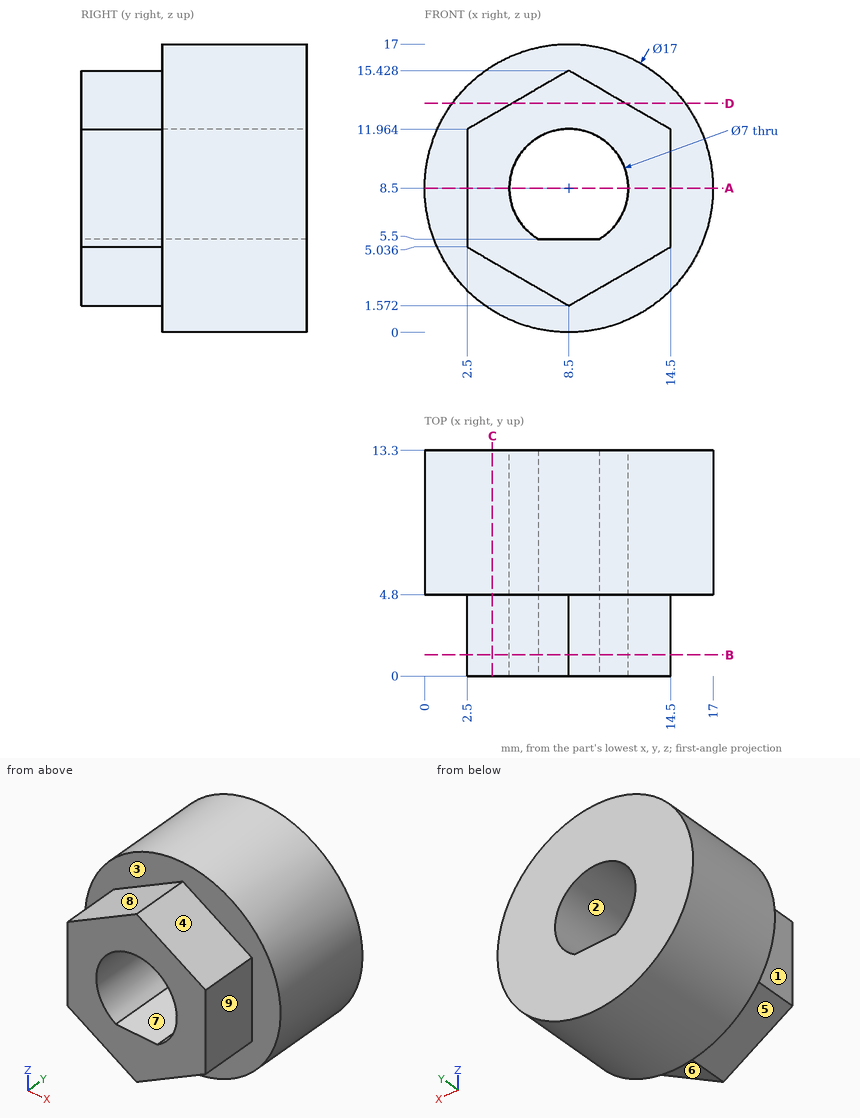
Study the drawing (mm; zero at the part's minimum x, y, z) and answer. A direction names the side the tool comes from. Coordinates: 2 decimals unless noted, no trailing zeros. Loops run counter-clockwise (first coordinate to the right, second up) from the corner with the lowest first, then second, coordinate; pieces in that order, holes last. Notation, with made-up numbers: (55, 85.5) -> (66, 85.5) arc R21 cw to (66, 120.5) -> close; hole circle Ø7 at (0.5, 19). An arc over 180 degrees is marked (long way). Write each question's results on one line, items separated by ' | '. Start each with the question number.
1) Find section C-C on x = 4. Determine the outline of the cut face in (y, z).
2) Find section B-B on y = 1.25. Determine the outline of the cut face in (x, z).
3) Find section D-D on z = 13.5. Determine the outline of the cut face in (x, y), then the cut area to 3 significant figures.
4) Flat-ended cylindrical pins translate along their axes: P1, Ø1.4, axis at y = 3, z = 8, coming from the -X side; P2, Ø1.4, axis at y = 2.5, z = 9.5, coming from the +X side; P3, Ø5, axis at y = 5.5, z = 15, coming from the -X side. Find the tip coordinate at first contact, or state that the pin passes through.
5) The mould has two halves that part along X. Classify the marked faces 1, 2, 3 and 4: pulls with the +X half, pulls with the -X half, needs draft (parallel to the pull), parting line crosses it, or undercut.
6) For the marked faces 5, 6, 7, 8 and 9, determine the directions among +Z, -Z, +X, -X, +Y, -Y from which every point of the face is accessible in a straight line to the end or side of a thin tool.
7) Find section A-A on z = 8.5. Determine the outline of the cut face in (x, y).
8) Consider line 1 along X through (y, z) = (3, 8.5); line 2 along X through (y, z) = (7.5, 8.5); line 3 along Y through (x, z) = (4, 13.5). Determine where each line is inside the solid, lowest interval first.
Response values:
1) outline: (0, 4.17) -> (4.8, 4.17) -> (4.8, 1.29) -> (13.3, 1.29) -> (13.3, 15.71) -> (4.8, 15.71) -> (4.8, 12.83) -> (0, 12.83) -> close
2) outline: (2.5, 5.04) -> (8.5, 1.57) -> (14.5, 5.04) -> (14.5, 11.96) -> (8.5, 15.43) -> (2.5, 11.96) -> close; hole (6.7, 5.5) -> (10.3, 5.5) arc R3.5 ccw (long way) to start
3) outline: (1.63, 4.8) -> (5.16, 4.8) -> (5.16, 0) -> (11.84, 0) -> (11.84, 4.8) -> (15.37, 4.8) -> (15.37, 13.3) -> (1.63, 13.3) -> close | area: 149 mm^2
4) P1: stops at x = 2.5 | P2: stops at x = 14.5 | P3: stops at x = 1
5) face 1: pulls with the -X half | face 2: undercut | face 3: needs draft | face 4: pulls with the +X half
6) face 5: -Z, -X, -Y | face 6: -Z, +X, -Y | face 7: +Y, -Y | face 8: +Z, -X, -Y | face 9: +Z, -Z, +X, -Y
7) outline: (0, 4.8) -> (2.5, 4.8) -> (2.5, 0) -> (5, 0) -> (5, 13.3) -> (0, 13.3) -> close; (12, 0) -> (14.5, 0) -> (14.5, 4.8) -> (17, 4.8) -> (17, 13.3) -> (12, 13.3) -> close
8) line 1: x = 2.5 to 5, 12 to 14.5 | line 2: x = 0 to 5, 12 to 17 | line 3: y = 4.8 to 13.3
